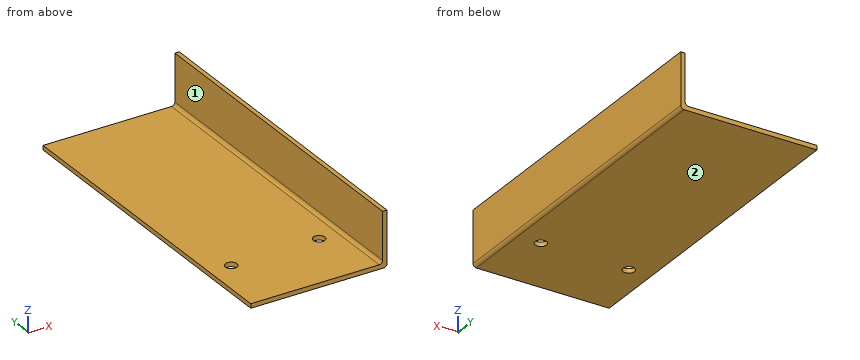
```python
from build123d import *

# Parameters (mm, degrees)
SKETCH1_W        = 120
SKETCH1_H        = 4
EXTRUDE_2_DEPTH  = 300
FILLET_2_R       = 3
HOLES_LEFT_REACH = 6
SKETCH3_R        = 5.25


with BuildPart() as part:
    # Sketch1 → Extrude 2 (new body)
    with BuildSketch(Plane(origin=(0, 0, 0), x_dir=(1, 0, 0), z_dir=(0, 1, 0))):
        Polygon((64, 2), (60, 2), (60, -2), (60, -48), (64, -48), align=None)
        Rectangle(SKETCH1_W, SKETCH1_H)
    extrude(amount=EXTRUDE_2_DEPTH)

    # Fillet 2
    fillet_2_edges = [part.edges().sort_by_distance(p)[0] for p in [
        (64, 150, -2),
        (60, 150, 2),
    ]]
    fillet(fillet_2_edges, radius=FILLET_2_R)

    # Sketch3 → Holes left (cut, up to next)
    with BuildSketch(Plane.XY.offset(2), mode=Mode.PRIVATE) as holes_left_sk1:
        with Locations((-40, 60)):
            Circle(SKETCH3_R)
    holes_left_tool1 = extrude(holes_left_sk1.sketch, amount=-HOLES_LEFT_REACH, mode=Mode.PRIVATE) & part.part
    add(holes_left_tool1.solids().sort_by_distance((-40, 60, 2))[0], mode=Mode.SUBTRACT)
    # Sketch3 → Holes left (cut, up to next)
    with BuildSketch(Plane.XY.offset(2), mode=Mode.PRIVATE) as holes_left_sk2:
        with Locations((40, 60)):
            Circle(SKETCH3_R)
    holes_left_tool2 = extrude(holes_left_sk2.sketch, amount=-HOLES_LEFT_REACH, mode=Mode.PRIVATE) & part.part
    add(holes_left_tool2.solids().sort_by_distance((40, 60, 2))[0], mode=Mode.SUBTRACT)


solid = part.part
```
Source: CAD feature listing. Evaluate the final solid. Frame: model axes, mm. Face numbers are marked on the shaded views. A direction names the side the tool comes from. Round coordinates to 2 decimals unless told otherwise and drop trailing zeros. Loops run counter-clockwise (first coordinate to the right, second up) from the corner with the lowest first, then second, coordinate; pieces in that order, holes last. Notation, with made-up numbers: (58, 38.25) - (109, 38.25) arc R26 ccw to (109, 75.25) - close; hole circle Ø10 at (16, -26.5). An arc over 180 degrees is marked (long way). Use CSV: the item, a comma, the result in double quotes.
Q1. Pin query (flat end, axial travel): pin 1 Ø6 at (y, z) = (152.5, 18.5) entering from -X; pin 2 Ø2 at (x, y) = (43.5, 133) entering from +Z. Return the tip coordinate at first contact, or that it passes through.
Reported:
pin 1,"x = 60"
pin 2,"z = 2"
Q2. Section query A-A, the plane y = 60. Output: boundary loops of the cut face in (x, z), then the cut area to 3 significant figures.
Reported:
outline,"(-60, -2) - (-45.25, -2) - (-45.25, 2) - (-60, 2) - close; (-34.75, -2) - (34.75, -2) - (34.75, 2) - (-34.75, 2) - close; (45.25, -2) - (61, -2) arc R3 ccw to (64, 1) - (64, 48) - (60, 48) - (60, 5) arc R3 cw to (57, 2) - (45.25, 2) - close"
area,"596 mm^2"
Q3. Section query D-D, the plane z = 32. Output: boundary loops of the cut face in (x, y).
Reported:
outline,"(60, 0) - (64, 0) - (64, 300) - (60, 300) - close"
Q4. Ray query, line 1 along Y through (x, z) = (40, 0.15); line 2 along Z through (x, y) = (54.5, 111); line 3 along X through (y, z) = (77.5, 12.5). Return the intervals inside material, ascending.
Reported:
line 1,"0 to 54.75, 65.25 to 300"
line 2,"-2 to 2"
line 3,"60 to 64"
Q5. Section query C-C, the plane y = 120. Output: boundary loops of the cut face in (x, z).
Reported:
outline,"(-60, -2) - (61, -2) arc R3 ccw to (64, 1) - (64, 48) - (60, 48) - (60, 5) arc R3 cw to (57, 2) - (-60, 2) - close"
Q6. Reachability of the marked faces 1 and 2 from +Z, -Z, +X, -X, +Y, -Y: full face, straight path, thin tool, end or side. Return the list, or none.
Reported:
face 1,"+Z, -X, +Y, -Y"
face 2,"-Z, +X, -X, +Y, -Y"
Q7. Section query B-B, the plane x = -40. Output: boundary loops of the cut face in (y, z).
Reported:
outline,"(0, -2) - (54.75, -2) - (54.75, 2) - (0, 2) - close; (65.25, -2) - (300, -2) - (300, 2) - (65.25, 2) - close"
